```python
from build123d import *

# Parameters (mm, degrees)
F1_DEPTH = 60
F2_DEPTH = 60
F4_D     = 3.2
F4_DEPTH = 10
F4_TIP   = 0.9613769904
F5_W     = 6.35
F5_H     = 6.35
F6_DEPTH = 25


with BuildPart() as f1:
    # F0 (on Top) → F1 (new body)
    with BuildSketch(Plane.XY):
        with BuildLine():
            ThreePointArc((-15.0151466486, -4.363634278), (-12.5045454624, 9.3878791946), (0, 15.636365722))
            Line((0, 15.636365722), (0, 17.5))
            ThreePointArc((0, 17.5), (-17.5, 0), (0, -17.5))
            Line((0, -17.5), (0, -15.636365722))
            ThreePointArc((0, -15.636365722), (-7.7954240269, -13.5546042817), (-13.5151466486, -7.863634278))
            ThreePointArc((-13.5151466486, -7.863634278), (-14.3720878409, -6.1594662175), (-15.0151466486, -4.363634278))
        make_face()
        with BuildLine():
            Line((0, 17.5), (0, 15.636365722))
            ThreePointArc((0, 15.636365722), (12.5045454624, 9.3878791946), (15.0151466486, -4.363634278))
            ThreePointArc((15.0151466486, -4.363634278), (14.3720878409, -6.1594662175), (13.5151466486, -7.863634278))
            ThreePointArc((13.5151466486, -7.863634278), (7.7954240269, -13.5546042817), (0, -15.636365722))
            Line((0, -15.636365722), (0, -17.5))
            ThreePointArc((0, -17.5), (17.5, 0), (0, 17.5))
        make_face()
    extrude(amount=F1_DEPTH)

    # F0 (on Top) → F2 (join)
    with BuildSketch(Plane.XY):
        with BuildLine():
            Line((-13.5151466486, -4.363634278), (-15.0151466486, -4.363634278))
            ThreePointArc((-15.0151466486, -4.363634278), (-14.3720878409, -6.1594662175), (-13.5151466486, -7.863634278))
            Line((-13.5151466486, -7.863634278), (-13.5151466486, -4.363634278))
        make_face()
        with BuildLine():
            ThreePointArc((13.5151466486, -7.863634278), (14.3720878409, -6.1594662175), (15.0151466486, -4.363634278))
            Line((15.0151466486, -4.363634278), (13.5151466486, -4.363634278))
            Line((13.5151466486, -4.363634278), (13.5151466486, -7.863634278))
        make_face()
    extrude(amount=F2_DEPTH)

    # F4
    with Locations(Plane.XY.offset(60)):
        with Locations((12, 12), (-12, 12), (-12, -12), (12, -12)):
            Hole(F4_D / 2, depth=F4_DEPTH)
            with Locations((0, 0, -(F4_DEPTH + F4_TIP / 2))):  # 118° drill point
                Cone(0, F4_D / 2, F4_TIP, mode=Mode.SUBTRACT)

    # F5 (on Front) → F6 (cut)
    with BuildSketch(Plane.XZ):
        with Locations((-3.175, 20)):
            Rectangle(F5_W, F5_H)
        with Locations((3.175, 20)):
            Rectangle(F5_W, F5_H)
        with Locations((-3.175, 45.4)):
            Rectangle(F5_W, F5_H)
        with Locations((3.175, 45.4)):
            Rectangle(F5_W, F5_H)
        with Locations((-3.175, 32.7)):
            Rectangle(F5_W, F5_H)
        with Locations((3.175, 32.7)):
            Rectangle(F5_W, F5_H)
    extrude(amount=-F6_DEPTH, mode=Mode.SUBTRACT)


solid = f1.part
```
Input: part model. Units: mm. Frame: model coordinates. A direction names the side the tool comes from. Give positions to 0.01 mm unless a question says otherwise; leave off trailing zeros. Order: outer loops, then holes, each group sorted by start corner. A loop starts at its lowest first (then second) coordinate and runs counter-clockwise, first axis right, second up. Notation, with made-up numbers: (19.25, 36.25) - (30.25, 36.25) arc R11 cw to (30.25, 42.25) - close; hole circle Ø8 at (46, 78). An arc over 180 degrees is marked (long way). Use a Markdown table: item, result.
(1) Pin query (flat end, axial travel): pin 1 (2 mm diameter, centred on y = 15, z = 32, fed in from -X); pin 2 (1.6 mm diameter, centred on x = -1, y = 15, fed in from +Z); pin 3 (1.5 mm diameter, centred on y = -13.5, z = 22.5, fed in from +X); pin 4 (0.6 mm diameter, centred on y = 16, z = 44, fed in from +X). Return the tip coordinate at first contact, or that it passes through.
Computed values:
| item | result |
|---|---|
| pin 1 | stops at x = -10.5 |
| pin 2 | stops at z = 60 |
| pin 3 | stops at x = 11.99 |
| pin 4 | stops at x = 7.73 |
(2) Access query for faces 1 (the flat face through (-6.35, 15, 20)), 2 (the flat face through (13.515, -6, 30)), 3 (the cylindrical face through (12.65, -10.54, 54.93)), 4 (the cylindrical face through (-12.65, 10.54, 54.93)). Directions: +Z, -Z, +X, -X, +Y, -Y. A direction counts if a zero-diameter tool reaches every point of the face in a straight line with its end or side. Return the directions, or none.
Computed values:
| item | result |
|---|---|
| face 1 | +Y |
| face 2 | +Z, -Z |
| face 3 | +Z, -Y |
| face 4 | +Z, +Y |
(3) Line query: line 1 (X direction, y = -7, z = 24); line 2 (Y direction, x = -5, z = 26.5); line 3 (Y direction, x = 9, z = 8). Output: solid intervals per line, ascending. Write a range as from..to.
Computed values:
| item | result |
|---|---|
| line 1 | x = -16.04..-13.52, 13.52..16.04 |
| line 2 | y = -16.77..-14.82, 14.82..16.77 |
| line 3 | y = -15.01..-12.79, 12.79..15.01 |
(4) Draft query along X for faces 5 (the cylindrical face through (-6.703, -16.166, 29.58)), 6 (the cylindrical face through (12.674, 10.549, 54.93)), 7 (the cylindrical face through (10.54, 12.65, 54.93)). Return one class per face: released by +X, released by -X, zero draft, split by the parting line, or undercut.
Computed values:
| item | result |
|---|---|
| face 5 | split by the parting line |
| face 6 | undercut |
| face 7 | released by +X |
(5) Section query B-B (z = 40). Output: boundary loops of the cut face in (x, y), then the cut area to 3 significant figures.
Computed values:
| item | result |
|---|---|
| outline | circle Ø35 at (0, 0); hole (-15.02, -4.36) - (-13.52, -4.36) - (-13.52, -7.86) arc R15.64 ccw to (13.52, -7.86) - (13.52, -4.36) - (15.02, -4.36) arc R15.64 ccw (long way) to start |
| area | 200 mm2 |
(6) Section query C-C (x = 4). Output: boundary loops of the cut face in (y, z) (3 decimals), then the cut area to 3 significant figures.
Computed values:
| item | result |
|---|---|
| outline | (-17.037, 0) - (-15.116, 0) - (-15.116, 60) - (-17.037, 60) - close; (15.116, 0) - (17.037, 0) - (17.037, 16.825) - (15.116, 16.825) - close; (15.116, 23.175) - (17.037, 23.175) - (17.037, 29.525) - (15.116, 29.525) - close; (15.116, 35.875) - (17.037, 35.875) - (17.037, 42.225) - (15.116, 42.225) - close; (15.116, 48.575) - (17.037, 48.575) - (17.037, 60) - (15.116, 60) - close |
| area | 194 mm2 |
(7) Section query A-A (y = 0). Output: boundary loops of the cut face in (x, z).
Computed values:
| item | result |
|---|---|
| outline | (-17.5, 0) - (-15.64, 0) - (-15.64, 60) - (-17.5, 60) - close; (15.64, 0) - (17.5, 0) - (17.5, 60) - (15.64, 60) - close |
(8) Section query D-D (z = 31.5). Output: boundary loops of the cut face in (x, y), then the cut area to 3 significant figures.
Computed values:
| item | result |
|---|---|
| outline | (-15.02, -4.36) arc R15.64 cw to (-6.35, 14.29) - (-6.35, 16.31) arc R17.5 ccw (long way) to (6.35, 16.31) - (6.35, 14.29) arc R15.64 cw to (15.02, -4.36) - (13.52, -4.36) - (13.52, -7.86) arc R15.64 cw to (-13.52, -7.86) - (-13.52, -4.36) - close |
| area | 176 mm2 |
